Part model, mm, in its own coordinate system. A direction names the side the tool comes from. Coordinates: 2 decimals unless noted, no trailing zeros. Write each loop counter-clockwise with the first axis right and the second up, starting at its lowest first coordinate (ties: lowest second). Pieces come first, ordered by that corner, then holes. Notation, with made-up numbers: (-20.5, 71.25) -> (38.5, 71.25) arc R19 cw to (38.5, 92.25) -> close; hole circle Ø6 at (27.5, 66.5). An arc over 180 degrees is marked (long way). Write item = value, one per line. Start each with the question number.
Q1. Band-saw the part on B-B, the plane y = -7.25. List the corners of the cut face in (x, z).
Q2. Pull direction Z, two halves, no side cores. Call faces 1 (the flat face through (-0.2, -8.5, 93)), 2 (the cylindrical face through (5.89, -8.99, 94.57)), 3 (the flat face through (-15, -7, 94)): released by +Z, released by -Z, zero draft, split by the parting line, or undercut.
Q3. Pin check, flat tips, straight feed: P1, Ø2.5, axis at x = -5, z = 95, coming from the +Y side; P2, Ø1, axis at y = -9.5, z = 97.5, coming from the +X side. Stop position of each tip, or through.
Q4. Tool access for faces 4 (the flat face through (-9.99, -6.32, 95.58)), 5 (the conical face through (14.02, -9.41, 95.54)): list every direction of +Z, -Z, +X, -X, +Y, -Y with a clear straight run to the whole face (end or side of a thin tool).
Q5. Band-saw the part on D-D, the plane x = -5. List the corners of the cut face in (y, z).
Q6. Band-saw the part on C-C, the plane z = 96.65. List the corners of the cut face in (x, y), plus the area to 3 significant figures.
Q7. Band-saw the part on A-A, the plane x = 5.2. List the corners of the cut face in (y, z), plus the area to 3 significant figures.
Q8. Probe line 1 (Z direction, x = 5.2, y = -9.5); line 2 (X direction, y = -9.5, z = 95.9); line 3 (X direction, y = -9.05, z = 96.75). List the from-to ranges inside material, lowest first.
from build123d import *

# Parameters (mm, degrees)
BOX341_W           = 22
BOX341_H           = 4
BOX341_DEPTH       = 6
CHAMFER073_1_SIZE2 = 2.4
CHAMFER073_1_SIZE  = 5.9
CHAMFER073_2_SIZE2 = 2.4
CHAMFER073_2_SIZE  = 5.9
CYLINDER398_R      = 1.5
CYLINDER398_DEPTH  = 5
CYLINDER395_R      = 1.5
CYLINDER395_DEPTH  = 5
BOX342_W           = 30
BOX342_H           = 5.4
BOX342_DEPTH       = 5
CHAMFER074_1_SIZE2 = 2
CHAMFER074_1_SIZE  = 3
CHAMFER074_2_SIZE2 = 2
CHAMFER074_2_SIZE  = 3


with BuildPart() as cone008:
    # Cone007 → Cone007 (revolve)
    with BuildSketch(Plane(origin=(0, 0, 85), x_dir=(1, 0, 0), z_dir=(0, -1, 0))):
        Polygon((0, 0), (21, 0), (5, 41), (0, 41), align=None)
    revolve(axis=Axis((0, 0, 85), (0, 0, 1)))


with BuildPart() as chamfer096:
    # Box341 → Box341 (new body)
    with BuildSketch(Plane(origin=(-11, -8, 93), x_dir=(1, 0, 0), z_dir=(0, 0, 1))):
        with Locations((11, 2)):
            Rectangle(BOX341_W, BOX341_H)
    extrude(amount=BOX341_DEPTH)

    # Chamfer073 1
    chamfer073_1_edges = [chamfer096.edges().sort_by_distance(p)[0] for p in [
        (11, -6, 99),
    ]]
    chamfer073_1_side = chamfer096.faces().sort_by_distance((11, -6, 96))[0]
    chamfer(chamfer073_1_edges, length=CHAMFER073_1_SIZE, length2=CHAMFER073_1_SIZE2, reference=chamfer073_1_side)

    # Chamfer073 2
    chamfer073_2_edges = [chamfer096.edges().sort_by_distance(p)[0] for p in [
        (-11, -6, 99),
    ]]
    chamfer073_2_side = chamfer096.faces().sort_by_distance((-11, -6, 96))[0]
    chamfer(chamfer073_2_edges, length=CHAMFER073_2_SIZE, length2=CHAMFER073_2_SIZE2, reference=chamfer073_2_side)


with BuildPart() as cylinder398:
    # Cylinder398 → Cylinder398 (new body)
    with BuildSketch(Plane(origin=(5.2, -6, 95.9), x_dir=(1, 0, 0), z_dir=(0, -1, 0))):
        Circle(CYLINDER398_R)
    extrude(amount=CYLINDER398_DEPTH)


with BuildPart() as cut_out001:
    # Cylinder395 → Cylinder395 (new body)
    with BuildSketch(Plane(origin=(-5.8, -6, 95.9), x_dir=(1, 0, 0), z_dir=(0, -1, 0))):
        Circle(CYLINDER395_R)
    extrude(amount=CYLINDER395_DEPTH)

    # Compound201: union Cylinder398
    add(cylinder398.part)

    # Fusion087: union Chamfer096
    add(chamfer096.part)


with BuildPart() as obj1:
    # Box342 → Box342 (new body)
    with BuildSketch(Plane(origin=(-15, -10, 93), x_dir=(1, 0, 0), z_dir=(0, 0, 1))):
        with Locations((15, 2.7)):
            Rectangle(BOX342_W, BOX342_H)
    extrude(amount=BOX342_DEPTH)

    # Chamfer074 1
    chamfer074_1_edges = [obj1.edges().sort_by_distance(p)[0] for p in [
        (15, -7.3, 98),
    ]]
    chamfer074_1_side = obj1.faces().sort_by_distance((15, -7.3, 95.5))[0]
    chamfer(chamfer074_1_edges, length=CHAMFER074_1_SIZE, length2=CHAMFER074_1_SIZE2, reference=chamfer074_1_side)

    # Chamfer074 2
    chamfer074_2_edges = [obj1.edges().sort_by_distance(p)[0] for p in [
        (-15, -7.3, 98),
    ]]
    chamfer074_2_side = obj1.faces().sort_by_distance((-15, -7.3, 95.5))[0]
    chamfer(chamfer074_2_edges, length=CHAMFER074_2_SIZE, length2=CHAMFER074_2_SIZE2, reference=chamfer074_2_side)

    # Cut226: cut cut-out001
    add(cut_out001.part, mode=Mode.SUBTRACT)

    # Common007: intersect Cone008
    add(cone008.part, mode=Mode.INTERSECT)


solid = obj1.part
Ans:
q1.outline = (-15, 93) -> (-11, 93) -> (-11, 93.1) -> (-9.01, 98) -> (-13, 98) -> (-15, 95) -> close; (9.01, 98) -> (11, 93.1) -> (11, 93) -> (15, 93) -> (15, 95) -> (13, 98) -> close
q2.face_1 = released by -Z
q2.face_2 = undercut
q2.face_3 = zero draft
q3.P1 = -8
q3.P2 = 13.45
q4.face_4 = -Z, +Y
q4.face_5 = +Z, +X, -Y
q5.outline = (-10, 93) -> (-8, 93) -> (-8, 94.63) -> (-10, 94.63) -> close; (-10, 97.17) -> (-8, 97.17) -> (-8, 98) -> (-10, 98) -> close
q6.outline = (-13.9, -8.8) arc R16.45 ccw to (-13.07, -10) -> (-7.1, -10) -> (-7.1, -8) -> (-9.56, -8) -> (-9.56, -4.6) -> (-13.9, -4.6) -> close; (-4.5, -10) -> (3.9, -10) -> (3.9, -8) -> (-4.5, -8) -> close; (6.5, -10) -> (13.07, -10) arc R16.45 ccw to (13.9, -8.8) -> (13.9, -4.6) -> (9.56, -4.6) -> (9.56, -8) -> (6.5, -8) -> close
q6.area = 73.8 mm2
q7.outline = (-10, 93) -> (-8, 93) -> (-8, 94.4) -> (-10, 94.4) -> close; (-10, 97.4) -> (-8, 97.4) -> (-8, 98) -> (-10, 98) -> close
q7.area = 4.00 mm2
q8.line_1 = 93 to 94.4, 97.4 to 98
q8.line_2 = -13.79 to -7.3, -4.3 to 3.7, 6.7 to 13.79
q8.line_3 = -13.69 to -7.04, -4.56 to 3.96, 6.44 to 13.69
